Read the model definition and answer for the solid it produces. Units are mm, in the model's axes. A direction names the side the tool comes from. Round coordinates to 2 decimals unless told otherwise and drop trailing zeros. Loops run counter-clockwise (first coordinate to the right, second up) from the corner with the lowest first, then second, coordinate; pieces in that order, holes last. Notation, with made-up numbers: M -11.5,-5.5 L 36.5,-5.5 A12 cw 36.5,11.5 Z; hole C -15,88.25 d11. An arc over 180 degrees is marked long. Write each question's results on one line, items separated by ' | '.
```python
from build123d import *

# Parameters (mm, degrees)
SKETCH1_W            = 217.17
SKETCH1_H            = 49.022
BOSS_EXTRUDE1_DEPTH  = 6.35
SKETCH5_W            = 20.066
SKETCH5_H            = 25.4
BOSS_EXTRUDE3_DEPTH  = 6.35
SKETCH6_W            = 25.4
SKETCH6_H            = 20.066
BOSS_EXTRUDE4_DEPTH  = 6.35
SKETCH7_R            = 1.75
CUT_EXTRUDE1_DEPTH   = 119.914732704
SKETCH9_R            = 2.286
CUT_EXTRUDE2_DEPTH   = 119.213807607
BOSS_EXTRUDE8_DEPTH  = 3.175
BOSS_EXTRUDE9_START  = 1.2
SKETCH15_R           = 6.35
SKETCH15_R_2         = 1.75
BOSS_EXTRUDE9_DEPTH  = 1.2
CUT_EXTRUDE4_START   = -3.175
SKETCH16_R           = 6.35
CUT_EXTRUDE4_DEPTH   = 3.175
SKETCH17_R           = 8.255
CUT_EXTRUDE5_DEPTH   = 119.914732704
SKETCH18_W           = 33.319
SKETCH18_H           = 20.066
BOSS_EXTRUDE10_DEPTH = 6.35
SKETCH19_R           = 2.286
BOSS_EXTRUDE11_DEPTH = 6.35
BOSS_EXTRUDE12_START = 6.35
SKETCH20_W           = 26.416
SKETCH20_H           = 19.05
SKETCH20_R           = 2.286
BOSS_EXTRUDE12_DEPTH = 6.35
BOSS_EXTRUDE13_DEPTH = 3.175
BOSS_EXTRUDE14_DEPTH = 3.175
BOSS_EXTRUDE15_DEPTH = 6.35
BOSS_EXTRUDE16_DEPTH = 6.35
FILLET2_R            = 6.35
FILLET3_R            = 6.35


with BuildPart() as part:
    # Sketch1 → Boss-Extrude1 (new body)
    with BuildSketch(Plane(origin=(0, 0, 0), x_dir=(1, 0, 0), z_dir=(0, 1, 0))):
        Rectangle(SKETCH1_W, SKETCH1_H)
    extrude(amount=BOSS_EXTRUDE1_DEPTH)

    # Sketch5 → Boss-Extrude3 (add)
    with BuildSketch(Plane.XY.offset(24.511)):
        with Locations((-98.552, -6.35)):
            Rectangle(SKETCH5_W, SKETCH5_H)
        with Locations((98.552, -6.35)):
            Rectangle(SKETCH5_W, SKETCH5_H)
    extrude(amount=-BOSS_EXTRUDE3_DEPTH)

    # Sketch6 → Boss-Extrude4 (add)
    with BuildSketch(Plane(origin=(0, 0, 0), x_dir=(-1, 0, 0), z_dir=(0, -1, 0))):
        with Locations((42.5, -34.544)):
            Rectangle(SKETCH6_W, SKETCH6_H)
        with Locations((-42.5, -34.544)):
            Rectangle(SKETCH6_W, SKETCH6_H)
    extrude(amount=-BOSS_EXTRUDE4_DEPTH)

    # Sketch7 → Cut-Extrude1 (cut, through all)
    with BuildSketch(Plane.XZ):
        with Locations(Location((-42.5, 34.544, 0), (0, 0, 270))):
            Circle(SKETCH7_R)
        with Locations(Location((42.5, 34.544, 0), (0, 0, 270))):
            Circle(SKETCH7_R)
    extrude(amount=-CUT_EXTRUDE1_DEPTH, mode=Mode.SUBTRACT)

    # Sketch9 → Cut-Extrude2 (cut, through all)
    with BuildSketch(Plane(origin=(0, 0, 18.161), x_dir=(-1, 0, 0), z_dir=(0, 0, -1))):
        with Locations((98.552, -9.525)):
            Circle(SKETCH9_R)
        with Locations((-98.552, -9.525)):
            Circle(SKETCH9_R)
    extrude(amount=-CUT_EXTRUDE2_DEPTH, mode=Mode.SUBTRACT)

    # Sketch14 → Boss-Extrude8 (add)
    with BuildSketch(Plane.ZY.offset(108.585)):
        Polygon((-24.511, 6.35), (-24.511, 0), (18.161, 0), (18.161, -19.05), (24.511, -19.05), (24.511, 6.35), align=None)
    extrude(amount=-BOSS_EXTRUDE8_DEPTH)

    # Sketch15 → Boss-Extrude9 (add)
    # profile 1 of 2: a face of its own
    with BuildSketch(Plane.XZ.offset(BOSS_EXTRUDE9_START)):
        with Locations(Location((42.5, 34.544, 0), (0, 0, 270))):
            Circle(SKETCH15_R)
        with Locations(Location((42.5, 34.544, 0), (0, 0, 270))):
            Circle(SKETCH15_R_2, mode=Mode.SUBTRACT)
    # profile 2 of 2: a face of its own
    with BuildSketch(Plane.XZ.offset(BOSS_EXTRUDE9_START)):
        with Locations(Location((-42.5, 34.544, 0), (0, 0, 270))):
            Circle(SKETCH15_R)
        with Locations(Location((-42.5, 34.544, 0), (0, 0, 270))):
            Circle(SKETCH15_R_2, mode=Mode.SUBTRACT)
    extrude(amount=-BOSS_EXTRUDE9_DEPTH)

    # Sketch16 → Cut-Extrude4 (cut)
    with BuildSketch(Plane(origin=(0, 6.35, 0), x_dir=(1, 0, 0), z_dir=(0, 1, 0)).offset(CUT_EXTRUDE4_START)):
        with Locations(Location((42.5, -34.544, 0), (0, 0, 90))):
            Circle(SKETCH16_R)
        with Locations(Location((-42.5, -34.544, 0), (0, 0, 90))):
            Circle(SKETCH16_R)
    extrude(amount=CUT_EXTRUDE4_DEPTH, mode=Mode.SUBTRACT)

    # Sketch17 → Cut-Extrude5 (cut, through all)
    with BuildSketch(Plane.XZ):
        with Locations(Location((-45.675, -12.956, 0), (0, 0, 270))):
            Circle(SKETCH17_R)
        with Locations(Location((45.675, -12.956, 0), (0, 0, 270))):
            Circle(SKETCH17_R)
    extrude(amount=-CUT_EXTRUDE5_DEPTH, mode=Mode.SUBTRACT)

    # Sketch18 → Boss-Extrude10 (add)
    with BuildSketch(Plane.XZ):
        with Locations((71.8595, 34.544)):
            Rectangle(SKETCH18_W, SKETCH18_H)
        with Locations((-71.8595, 34.544)):
            Rectangle(SKETCH18_W, SKETCH18_H)
    extrude(amount=-BOSS_EXTRUDE10_DEPTH)

    # Sketch19 → Boss-Extrude11 (add)
    with BuildSketch(Plane.ZY.offset(-88.519)):
        Polygon((24.511, -19.05), (44.577, -19.05), (44.577, 0), (24.511, 0), (18.161, 0), (18.161, -19.05), align=None)
        with Locations((34.544, -9.525)):
            Circle(SKETCH19_R, mode=Mode.SUBTRACT)
    extrude(amount=BOSS_EXTRUDE11_DEPTH)

    # Sketch20 → Boss-Extrude12 (add)
    with BuildSketch(Plane(origin=(-88.519, 0, 0), x_dir=(0, 0, -1), z_dir=(1, 0, 0)).offset(BOSS_EXTRUDE12_START)):
        with Locations((-31.369, -9.525)):
            Rectangle(SKETCH20_W, SKETCH20_H)
        with Locations(Location((-34.544, -9.525, 0), (0, 0, 180))):
            Circle(SKETCH20_R, mode=Mode.SUBTRACT)
    extrude(amount=-BOSS_EXTRUDE12_DEPTH)

    # Sketch21 → Boss-Extrude13 (add)
    with BuildSketch(Plane.ZY.offset(108.585)):
        Polygon((18.161, -19.05), (-0.889, 0), (18.161, 0), align=None)
    extrude(amount=-BOSS_EXTRUDE13_DEPTH)

    # Sketch22 → Boss-Extrude14 (add)
    with BuildSketch(Plane(origin=(108.585, 0, 0), x_dir=(0, 0, -1), z_dir=(1, 0, 0))):
        Polygon((-18.161, 0), (-18.161, -19.05), (0.889, 0), align=None)
    extrude(amount=-BOSS_EXTRUDE14_DEPTH)

    # Sketch23 → Boss-Extrude15 (add)
    with BuildSketch(Plane(origin=(-82.169, 0, 0), x_dir=(0, 0, -1), z_dir=(1, 0, 0))):
        Polygon((-18.161, 0), (-18.161, -19.05), (0.889, 0), align=None)
    extrude(amount=-BOSS_EXTRUDE15_DEPTH)

    # Sketch24 → Boss-Extrude16 (add)
    with BuildSketch(Plane.ZY.offset(-82.169)):
        Polygon((18.161, 0), (-0.889, 0), (18.161, -19.05), align=None)
    extrude(amount=-BOSS_EXTRUDE16_DEPTH)

    # Fillet2
    fillet2_edges = [part.edges().sort_by_distance(p)[0] for p in [
        (85.344, -19.05, 44.577),
        (-85.344, -19.05, 44.577),
        (-29.8, 3.175, 44.577),
        (-29.8, 3.175, 24.511),
        (29.8, 3.175, 24.511),
        (29.8, 3.175, 44.577),
    ]]
    fillet(fillet2_edges, radius=FILLET2_R)

    # Fillet3
    # the kernel refuses this fillet: 6.35 mm, written as the material it adds along each edge
    with BuildSketch(Plane(origin=(-108.585, 0, -0.889), x_dir=(0, 0, -1), z_dir=(1, 0, 0))) as fillet3_piece_1:
        with BuildLine():
            CenterArc((FILLET3_R * 0.414213562373, -FILLET3_R), FILLET3_R, 90, 45)
            Line((-FILLET3_R * 0.292893218813, -FILLET3_R * 0.292893218813), (0, 0))
            Line((0, 0), (FILLET3_R * 0.414213562373, 0))
        make_face()
    extrude(amount=3.175)
    with BuildSketch(Plane(origin=(108.585, 0, -0.889), x_dir=(0, 0, -1), z_dir=(-1, 0, 0))) as fillet3_piece_2:
        with BuildLine():
            CenterArc((FILLET3_R * 0.414213562373, FILLET3_R), FILLET3_R, 225, 45)
            Line((-FILLET3_R * 0.292893218813, FILLET3_R * 0.292893218813), (0, 0))
            Line((0, 0), (FILLET3_R * 0.414213562373, 0))
        make_face()
    extrude(amount=3.175)
    with BuildSketch(Plane(origin=(-82.169, 0, -0.889), x_dir=(0, 0, -1), z_dir=(-1, 0, 0))) as fillet3_piece_3:
        with BuildLine():
            CenterArc((FILLET3_R * 0.414213562373, FILLET3_R), FILLET3_R, 225, 45)
            Line((-FILLET3_R * 0.292893218813, FILLET3_R * 0.292893218813), (0, 0))
            Line((0, 0), (FILLET3_R * 0.414213562373, 0))
        make_face()
    extrude(amount=6.35)
    with BuildSketch(Plane(origin=(82.169, 0, -0.889), x_dir=(0, 0, -1), z_dir=(1, 0, 0))) as fillet3_piece_4:
        with BuildLine():
            CenterArc((FILLET3_R * 0.414213562373, -FILLET3_R), FILLET3_R, 90, 45)
            Line((-FILLET3_R * 0.292893218813, -FILLET3_R * 0.292893218813), (0, 0))
            Line((0, 0), (FILLET3_R * 0.414213562373, 0))
        make_face()
    extrude(amount=6.35)
    # the kernel refuses this fillet: 6.35 mm, written as the material it takes off along each edge
    with BuildSketch(Plane(origin=(-108.585, -19.05, 40.386), x_dir=(1, 0, 0), z_dir=(0, 0, -1))) as fillet3_2_piece_1:
        with BuildLine():
            CenterArc((FILLET3_R, -FILLET3_R), FILLET3_R, 90, 90)
            Line((0, -FILLET3_R), (0, 0))
            Line((0, 0), (FILLET3_R, 0))
        make_face()
    extrude(amount=38.1, mode=Mode.SUBTRACT)
    with BuildSketch(Plane(origin=(108.585, -19.05, 40.386), x_dir=(-1, 0, 0), z_dir=(0, 0, -1)), Plane(origin=(-108.585, -15.875, -24.511), x_dir=(0, 0, 1), z_dir=(0, 1, 0)), Plane(origin=(108.585, -15.875, -24.511), x_dir=(-1, 0, 0), z_dir=(0, 1, 0))) as fillet3_2_piece_2:
        with BuildLine():
            CenterArc((FILLET3_R, FILLET3_R), FILLET3_R, 180, 90)
            Line((0, FILLET3_R), (0, 0))
            Line((0, 0), (FILLET3_R, 0))
        make_face()
    extrude(amount=38.1, mode=Mode.SUBTRACT)


solid = part.part
```
1. Determine the mould class of faces 1 (the face through (-29.8, 3, 35)), 2 (the face through (51.25, 3.13, -6.87)), 3 (the face through (40.068, -0.608, 28.678)) for opening direction Z: released by +Z, released by -Z, zero draft, split by the parting line, or undercut.
Completed:
face 1: zero draft | face 2: undercut | face 3: split by the parting line
2. Find section B-B, the plane x = 1. Give the vertices of the cut face in (y, z).
Completed:
outline: M 0,-24.51 L 6.35,-24.51 L 6.35,24.51 L 0,24.51 Z
3. Find section C-C, the plane z = 5.5. Give the vertices of the cut face in (x, y) (3 decimals), then the cut area to 3 significant figures.
Completed:
outline: M -108.585,-6.389 L -105.41,-6.389 L -105.41,0 L -88.519,0 L -88.519,-6.389 L -82.169,-6.389 L -82.169,0 L 82.169,0 L 82.169,-6.389 L 88.519,-6.389 L 88.519,0 L 105.41,0 L 105.41,-6.389 L 108.585,-6.389 L 108.585,6.35 L -108.585,6.35 Z | area: 1,500 mm2
4. Which of the six approach directions +Z, -Z, +X, -X, +Y, -Y give full straight-line access (tool end or side, diameter ignored) to faces 4 (the face through (-40.59, -0.61, 28.49)), 5 (the face through (-41, 3.175, 33)), 6 (the face through (82.169, -9, 26)), 7 (the face through (98, -6, 24.511)), 8 (the face through (-88.519, -6, 35))?
Completed:
face 4: -Y | face 5: +Y | face 6: +Z, -Z, -Y | face 7: +Z, +X, +Y, -Y | face 8: +Z, -X, +Y, -Y
5. Find section A-A, the plane y = -15.5. Give the vertices of the cut face in (x, z), then the cut area to 3 significant figures.
Completed:
outline: M -107.93,14.61 L -105.41,14.61 L -105.41,18.16 L -88.52,18.16 L -88.52,14.61 L -82.17,14.61 L -82.17,43.93 L -88.52,43.93 L -88.52,24.51 L -107.93,24.51 Z; M 82.17,14.61 L 88.52,14.61 L 88.52,18.16 L 105.41,18.16 L 105.41,14.61 L 107.93,14.61 L 107.93,24.51 L 88.52,24.51 L 88.52,43.93 L 82.17,43.93 Z | area: 637 mm2
6. Find the intervals of material crossed by L1, parallel to X at y = -0.25, z = 8 (3 decimals); L2, parallel to X at y = -15, z = 25; L3, parallel to Y at x = -60, z = -14, in increasing order.
Completed:
L1: x = -108.585 to -105.41, -88.519 to -82.169, 82.169 to 88.519, 105.41 to 108.585 | L2: x = -88.52 to -82.17, 82.17 to 88.52 | L3: y = 0 to 6.35
7. Given P1, Ø21.5, axis at x = 45.675, z = -12.956, coming from the +Y side; P2, Ø7.5, axis at y = -9.525, z = 34.544, coming from the +X side; P3, Ø2, axis at x = 11, z = -17, coming from the -Y side; P4, Ø3, axis at y = 3, z = 36, coming from the -X side, each flat-ended and moving along its own axis, determine where each tip first touches the part or whether it passes through.
Completed:
P1: stops at y = 6.35 | P2: stops at x = 88.52 | P3: stops at y = 0 | P4: stops at x = -88.52
8. Find section D-D, the plane x = -74. Give the vertices of the cut face in (y, z), then the cut area to 3 significant figures.
Completed:
outline: M 0,-24.51 L 6.35,-24.51 L 6.35,44.58 L 0,44.58 Z | area: 439 mm2
